Build history of the part. All positions in model axes, mm. Round coordinates to 2 decimals unless told otherwise and drop trailing zeros. Write each loop counter-clockwise with the first axis right and the second up, starting at its lowest first coordinate (ties: lowest second). Pieces come first, ordered by that corner, then holes. Notation, with made-up numbers: (6, 52.5) -> (54, 52.5) arc R12 cw to (54, 75.5) -> close; hole circle Ø2 at (55, 80.25). An arc over 180 degrees is marked (long way). Answer in a Markdown table with one row per item. Add a question column.
from build123d import *

# Parameters (mm, degrees)
SKETCH1_R           = 35
BOSS_EXTRUDE1_DEPTH = 4
SKETCH2_R           = 1
SKETCH2_R_2         = 1.25
CUT_EXTRUDE1_DEPTH  = 50.658836072
CUT_EXTRUDE2_REACH  = 51.659
SKETCH3_R           = 4
SKETCH4_R           = 3
CUT_EXTRUDE3_DEPTH  = 2.5
SKETCH5_R           = 2
CUT_EXTRUDE4_DEPTH  = 2.5


with BuildPart() as part:
    # Sketch1 → Boss-Extrude1 (new body)
    with BuildSketch(Plane(origin=(0, 0, 0), x_dir=(1, 0, 0), z_dir=(0, 1, 0))):
        with Locations(Location((0, 0, 0), (0, 0, 270))):
            Circle(SKETCH1_R)
    extrude(amount=BOSS_EXTRUDE1_DEPTH)

    # Sketch2 → Cut-Extrude1 (cut, through all)
    with BuildSketch(Plane(origin=(0, 4, 0), x_dir=(1, 0, 0), z_dir=(0, 1, 0))):
        with Locations(Location((0, 8.227062517, 0), (0, 0, 270))):
            Circle(SKETCH2_R)
        with Locations(Location((8.227062517, 0, 0), (0, 0, 270))):
            Circle(SKETCH2_R)
        with Locations(Location((0, -8.227062517, 0), (0, 0, 270))):
            Circle(SKETCH2_R)
        with Locations(Location((-8.227062517, 0, 0), (0, 0, 270))):
            Circle(SKETCH2_R)
        with Locations(Location((0, -28, 0), (0, 0, 90))):
            Circle(SKETCH2_R_2)
        with Locations(Location((-24.248711306, 14, 0), (0, 0, 90))):
            Circle(SKETCH2_R_2)
        with Locations(Location((24.248711306, 14, 0), (0, 0, 90))):
            Circle(SKETCH2_R_2)
    extrude(amount=-CUT_EXTRUDE1_DEPTH, mode=Mode.SUBTRACT)

    # Sketch3 → Cut-Extrude2 (cut, up to next)
    with BuildSketch(Plane.XZ, mode=Mode.PRIVATE) as cut_extrude2_sk1:
        with Locations(Location((0, 0, 0), (0, 0, 270))):
            Circle(SKETCH3_R)
    cut_extrude2_tool1 = extrude(cut_extrude2_sk1.sketch, amount=-CUT_EXTRUDE2_REACH, mode=Mode.PRIVATE) & part.part
    add(cut_extrude2_tool1.solids().sort_by_distance((0, 0, 0))[0], mode=Mode.SUBTRACT)

    # Sketch4 → Cut-Extrude3 (cut)
    with BuildSketch(Plane(origin=(0, 4, 0), x_dir=(1, 0, 0), z_dir=(0, 1, 0))):
        with Locations(Location((24.248711306, 14, 0), (0, 0, 270))):
            Circle(SKETCH4_R)
        with Locations(Location((0, -28, 0), (0, 0, 270))):
            Circle(SKETCH4_R)
        with Locations(Location((-24.248711306, 14, 0), (0, 0, 270))):
            Circle(SKETCH4_R)
    extrude(amount=-CUT_EXTRUDE3_DEPTH, mode=Mode.SUBTRACT)

    # Sketch5 → Cut-Extrude4 (cut)
    with BuildSketch(Plane.XZ):
        with Locations(Location((0, 8.227062517, 0), (0, 0, 270))):
            Circle(SKETCH5_R)
        with Locations(Location((8.227062517, 0, 0), (0, 0, 270))):
            Circle(SKETCH5_R)
        with Locations(Location((0, -8.227062517, 0), (0, 0, 270))):
            Circle(SKETCH5_R)
        with Locations(Location((-8.227062517, 0, 0), (0, 0, 270))):
            Circle(SKETCH5_R)
    extrude(amount=-CUT_EXTRUDE4_DEPTH, mode=Mode.SUBTRACT)


solid = part.part
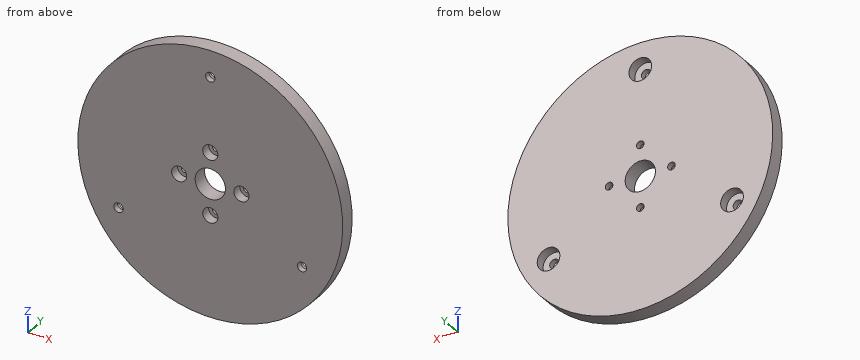
(1) Saw through at A-A (z = 0). List the corners of the cut face in (x, y), plus the area to 3 significant figures.
(2) Saw through at B-B (z = 28). List the corners of the cut face in (x, y).
(3) Saw through at C-C (z = -14). List the corners of the cut face in (x, y), plus the area to 3 significant figures.
(4) Saw through at D-D (z = 12). List the corners of the cut face in (x, y), plus the area to 3 significant figures.
(5) Probe line 1 along X through (y, z) = (0.7, 0); line 2 along X through (y, z) = (2.4, -14); line 3 along X through (y, z) = (0.3, -14). List the from-to ranges inside material, lowest first.
(6) Drop flat-ended pins along their axis: P1, Ø1.5, axis at x = 16, y = 3, coming from the -Z side; P2, Ø1.5, axis at x = -17.5, y = 3.5, coming from the -Z side; P3, Ø1.5, axis at y = 2.5, z = -10, coming from the -X side. Give the stop position or say it passes through.
Answer sheet:
| question | item | result |
|---|---|---|
| 1 | outline | (-35, 0) -> (-10.23, 0) -> (-10.23, 2.5) -> (-9.23, 2.5) -> (-9.23, 4) -> (-35, 4) -> close; (-7.23, 2.5) -> (-6.23, 2.5) -> (-6.23, 0) -> (-4, 0) -> (-4, 4) -> (-7.23, 4) -> close; (4, 0) -> (6.23, 0) -> (6.23, 2.5) -> (7.23, 2.5) -> (7.23, 4) -> (4, 4) -> close; (9.23, 2.5) -> (10.23, 2.5) -> (10.23, 0) -> (35, 0) -> (35, 4) -> (9.23, 4) -> close |
| 1 | area | 222 mm² |
| 2 | outline | (-21, 0) -> (-1.25, 0) -> (-1.25, 1.5) -> (-3, 1.5) -> (-3, 4) -> (-21, 4) -> close; (1.25, 0) -> (21, 0) -> (21, 4) -> (3, 4) -> (3, 1.5) -> (1.25, 1.5) -> close |
| 3 | outline | (-32.08, 0) -> (-25.5, 0) -> (-25.5, 1.5) -> (-27.25, 1.5) -> (-27.25, 4) -> (-32.08, 4) -> close; (-23, 0) -> (23, 0) -> (23, 1.5) -> (21.25, 1.5) -> (21.25, 4) -> (-21.25, 4) -> (-21.25, 1.5) -> (-23, 1.5) -> close; (25.5, 0) -> (32.08, 0) -> (32.08, 4) -> (27.25, 4) -> (27.25, 1.5) -> (25.5, 1.5) -> close |
| 3 | area | 219 mm² |
| 4 | outline | (-32.88, 0) -> (32.88, 0) -> (32.88, 4) -> (-32.88, 4) -> close |
| 4 | area | 263 mm² |
| 5 | line 1 | x = -35 to -10.23, -6.23 to -4, 4 to 6.23, 10.23 to 35 |
| 5 | line 2 | x = -32.08 to -27.25, -21.25 to 21.25, 27.25 to 32.08 |
| 5 | line 3 | x = -32.08 to -25.5, -23 to 23, 25.5 to 32.08 |
| 6 | P1 | stops at z = -31.5 |
| 6 | P2 | stops at z = -30.73 |
| 6 | P3 | stops at x = -33.76 |
